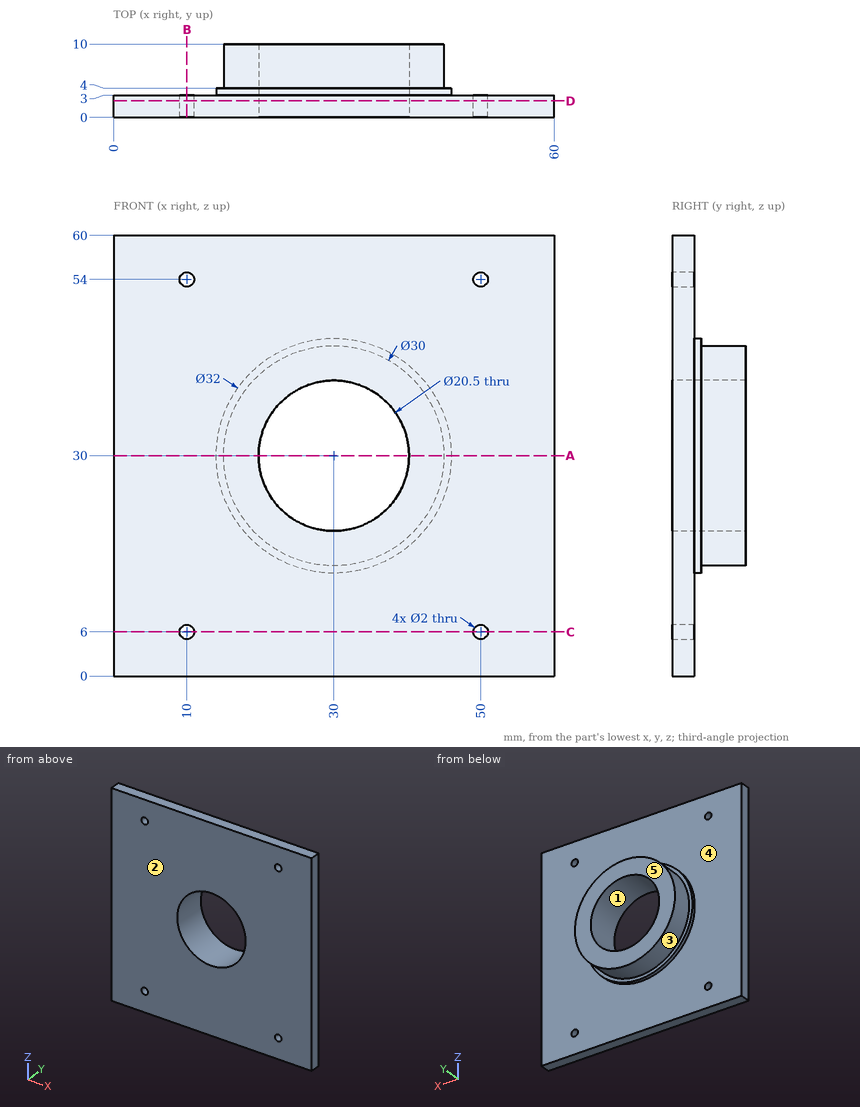
Drawing for the job (mm, zero at the part's lowest x, y, z). A direction names the side the tool comes from. Round coordinates to 2 decimals unless told otherwise and drop trailing zeros. Order: outer loops, then holes, each group sorted by start corner. A loop starts at its lowest first (then second) coordinate and runs counter-clockwise, first axis right, second up.
Item 1: Probe line 1 along Z through (x, y) = (50, 1.5); line 2 along X through (y, z) = (2.4, 6); line 3 along X through (y, z) = (4.75, 30). List the from-to ranges inside material, lowest first.
Item 2: Tool access for the marked faces 4 and 5: list every direction of +Z, -Z, +X, -X, +Y, -Y with a clear straight run to the whole face (end or side of a thin tool).
Item 3: Saw through at B-B on x = 10. Write the cut outline in (y, z).
Item 4: Saw through at C-C on z = 6. Write the cut outline in (x, y).
Item 5: Saw through at D-D on y = 2.25. Write the cut outline in (x, z).
Item 6: Pin check, flat tip, straight feed: pin 1 (4 mm diameter, centred on x = 11, z = 43, fed in from +Y). Stop position of the tip, or through.
Item 7: Mould opens along X. For the marked faces 1, 2 and 3 say: pulls with the +X half, pulls with the -X half, needs draft (parallel to the pull), parting line crosses it, or undercut.
Item 8: Saw through at A-A on z = 30. Write the cut outline in (x, y).
Reported:
1. line 1: z = 0 to 5, 7 to 53, 55 to 60
1. line 2: x = 0 to 9, 11 to 49, 51 to 60
1. line 3: x = 15 to 19.75, 40.25 to 45
2. face 4: +Y
2. face 5: +Z, -Z, +X, -X, +Y
3. outline: (0, 0) - (3, 0) - (3, 5) - (0, 5) - close; (0, 7) - (3, 7) - (3, 53) - (0, 53) - close; (0, 55) - (3, 55) - (3, 60) - (0, 60) - close
4. outline: (0, 0) - (9, 0) - (9, 3) - (0, 3) - close; (11, 0) - (49, 0) - (49, 3) - (11, 3) - close; (51, 0) - (60, 0) - (60, 3) - (51, 3) - close
5. outline: (0, 0) - (60, 0) - (60, 60) - (0, 60) - close; hole circle Ø2 at (10, 6); hole circle Ø2 at (10, 54); hole circle Ø20.5 at (30, 30); hole circle Ø2 at (50, 6); hole circle Ø2 at (50, 54)
6. pin 1: stops at y = 3
7. face 1: undercut
7. face 2: needs draft
7. face 3: parting line crosses it
8. outline: (0, 0) - (19.75, 0) - (19.75, 10) - (15, 10) - (15, 4) - (14, 4) - (14, 3) - (0, 3) - close; (40.25, 0) - (60, 0) - (60, 3) - (46, 3) - (46, 4) - (45, 4) - (45, 10) - (40.25, 10) - close
